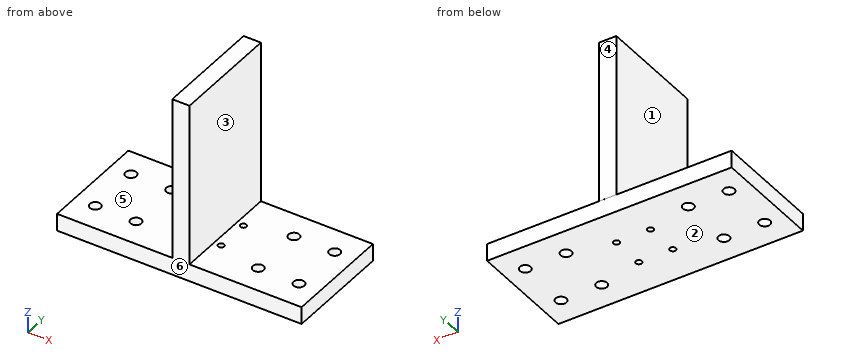
from build123d import *

# Parameters (mm, degrees)
CROQUIS1_W              = 180
CROQUIS1_H              = 80
CROQUIS1_R              = 4
CROQUIS1_R_2            = 2.25
SALIENTE_EXTRUIR1_DEPTH = 12.7
CROQUIS2_W              = 12.7
CROQUIS2_H              = 80.011204884
SALIENTE_EXTRUIR2_DEPTH = 120


with BuildPart() as part:
    # Croquis1 → Saliente-Extruir1 (new body)
    with BuildSketch(Plane.XY):
        with Locations((-60, 40)):
            Rectangle(CROQUIS1_W, CROQUIS1_H)
        with Locations((15, 20)):
            Circle(CROQUIS1_R, mode=Mode.SUBTRACT)
        with Locations((-15, 20)):
            Circle(CROQUIS1_R, mode=Mode.SUBTRACT)
        with Locations((15, 60)):
            Circle(CROQUIS1_R, mode=Mode.SUBTRACT)
        with Locations((-15, 60)):
            Circle(CROQUIS1_R, mode=Mode.SUBTRACT)
        with Locations((-105, 20)):
            Circle(CROQUIS1_R, mode=Mode.SUBTRACT)
        with Locations((-135, 20)):
            Circle(CROQUIS1_R, mode=Mode.SUBTRACT)
        with Locations((-135, 60)):
            Circle(CROQUIS1_R, mode=Mode.SUBTRACT)
        with Locations((-105, 60)):
            Circle(CROQUIS1_R, mode=Mode.SUBTRACT)
        with Locations((-72.288485416, 27.5)):
            Circle(CROQUIS1_R_2, mode=Mode.SUBTRACT)
        with Locations((-72.288485416, 52.5)):
            Circle(CROQUIS1_R_2, mode=Mode.SUBTRACT)
        with Locations((-47.288485416, 52.5)):
            Circle(CROQUIS1_R_2, mode=Mode.SUBTRACT)
        with Locations((-47.288485416, 27.5)):
            Circle(CROQUIS1_R_2, mode=Mode.SUBTRACT)
    extrude(amount=SALIENTE_EXTRUIR1_DEPTH)

    # Croquis2 → Saliente-Extruir2 (add)
    with BuildSketch(Plane.XY.offset(12.7)):
        with Locations((-58.85, 40.005602442)):
            Rectangle(CROQUIS2_W, CROQUIS2_H)
    extrude(amount=SALIENTE_EXTRUIR2_DEPTH)


solid = part.part
Work out the finished part from the listing and answer in its coordinate system (mm). Face numbers are marked on the shaded views. A direction names the side the tool comes from. Coordinates: 2 decimals unless noted, no trailing zeros. Write each loop counter-clockwise with the first axis right and the second up, starting at its lowest first coordinate (ties: lowest second). Pieces come first, ordered by that corner, then holes. Notation, with made-up numbers: M 52.25,-35.75 L 99.25,-35.75 A19 ccw 99.25,1.25 Z; hole C 3,-6 d11. An arc over 180 degrees is marked long. Answer as CSV lines item,"result". Start each with the question number.
Item 1: Determine the mould class of the marked faces 4, 5 and 6 for opening direction Y: released by +Y, released by -Y, zero draft, split by the parting line, or undercut.
Item 2: A tool of negligible diameter and unlimited length cuts with its end or side. For the marked faces 1, 2 and 3, from which of +Z, -Z, +X, -X, +Y, -Y can it reach the whole face along a straight path? Write none if from no direction.
Item 3: Section C-C on x = -21 is taken. Write down the section's boundary in (y, z), and give its area (3 significant figures).
Item 4: Section B-B on x = -105 is taken. Write down the section's boundary in (y, z), and give its area (3 significant figures).
Item 5: Section D-D on z = 53 is taken. Write down the section's boundary in (x, y).
Item 6: Consider L1, parallel to Y at x = -135, z = 8; L2, parallel to Z at x = -1, y = 55.5; L3, parallel to Y at x = -68, z = 8. Determine where each line is inside the solid, lowest interval first.
Item 7: Flat-ended cylindrical pins translate along their axes: P1, Ø13, axis at x = 15, y = 60, coming from the +Z side; P2, Ø10, axis at y = 15.5, z = 109.5, coming from the +X side; P3, Ø4, axis at x = -64, z = 7, coming from the +Y side; P4, Ø1, axis at x = -23.5, y = 40, coming from the -Z side. Find the tip coordinate at first contact, or state that the pin passes through.
Item 8: Section A-A on y = 20 is taken. Write down the section's boundary in (x, z).
Checks:
1,face 4,"released by +Y"
1,face 5,"zero draft"
1,face 6,"released by -Y"
2,face 1,"+Z, -X, +Y, -Y"
2,face 2,"-Z, +X, -X, +Y, -Y"
2,face 3,"+Z, +X, +Y, -Y"
3,outline,"M 0,0 L 80,0 L 80,12.7 L 0,12.7 Z"
3,area,"1,020 mm²"
4,outline,"M 0,0 L 16,0 L 16,12.7 L 0,12.7 Z; M 24,0 L 56,0 L 56,12.7 L 24,12.7 Z; M 64,0 L 80,0 L 80,12.7 L 64,12.7 Z"
4,area,"813 mm²"
5,outline,"M -65.2,0 L -52.5,0 L -52.5,80.01 L -65.2,80.01 Z"
6,L1,"y = 0 to 16, 24 to 56, 64 to 80"
6,L2,"z = 0 to 12.7"
6,L3,"y = 0 to 80"
7,P1,"stops at z = 12.7"
7,P2,"stops at x = -52.5"
7,P3,"stops at y = 80"
7,P4,"stops at z = 0"
8,outline,"M -150,0 L -139,0 L -139,12.7 L -150,12.7 Z; M -131,0 L -109,0 L -109,12.7 L -131,12.7 Z; M -101,0 L -19,0 L -19,12.7 L -52.5,12.7 L -52.5,132.7 L -65.2,132.7 L -65.2,12.7 L -101,12.7 Z; M -11,0 L 11,0 L 11,12.7 L -11,12.7 Z; M 19,0 L 30,0 L 30,12.7 L 19,12.7 Z"
